Can you work these out from the drawing? Everything is in mm from the part's minimum corner. Coordinates: 2 decimals unless noted, no trailing zeros. Loops run counter-clockwise (first coordinate to the right, second up) from the corner with the lowest first, then second, coordinate; pieces in that order, holes last.
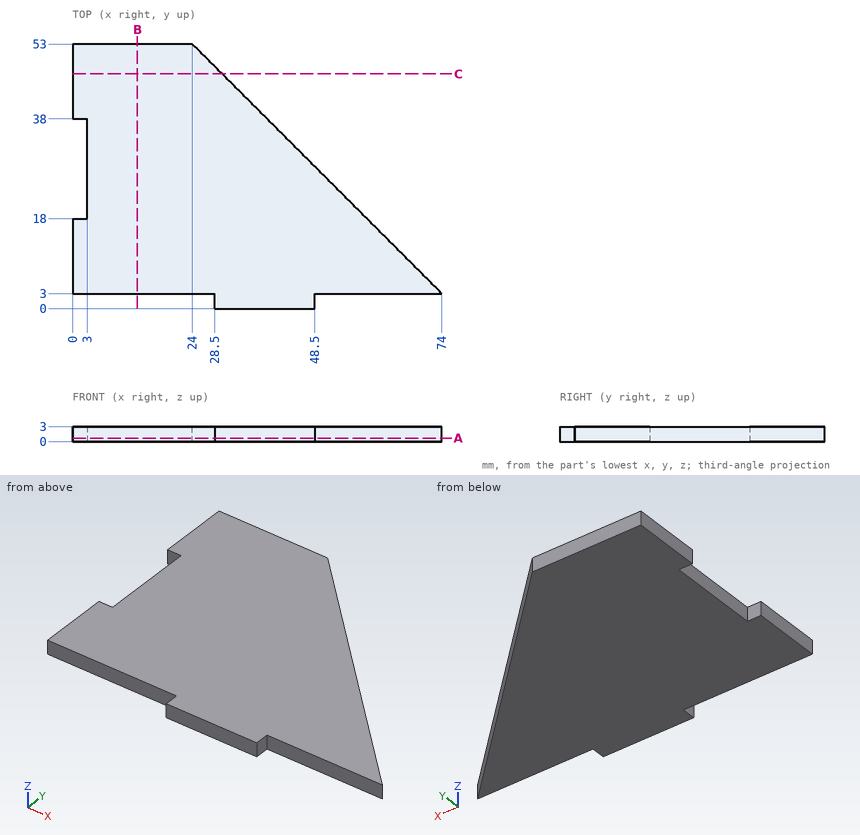
Item 1: Suppose I cut it at B-B, the plane x = 13. Please give me the cut outline in (y, z).
Results are:
outline: (3, 0) - (53, 0) - (53, 3) - (3, 3) - close
Item 2: Suppose I cut it at C-C, the plane y = 47. Please give me the cut outline in (x, z).
Results are:
outline: (0, 0) - (30, 0) - (30, 3) - (0, 3) - close
Item 3: Suppose I cut it at A-A, the plane z = 0.7. Please give me the cut outline in (x, y).
Results are:
outline: (0, 3) - (28.5, 3) - (28.5, 0) - (48.5, 0) - (48.5, 3) - (74, 3) - (24, 53) - (0, 53) - (0, 38) - (3, 38) - (3, 18) - (0, 18) - close
Item 4: I need wall thicknesses on line 1 along Y through (x, z) = (22, 0.8); line 2 along X through (y, z) = (2, 1.5); line 3 along X through (y, z) = (42, 2.4). Which ranges of each line are inside material? Lowest first, please.
Results are:
line 1: y = 3 to 53
line 2: x = 28.5 to 48.5
line 3: x = 0 to 35
Item 5: I'm going to push flat-ended pins straight in: P1, Ø1.5, axis at x = 1.5, z = 1, coming from the -Y side; P2, Ø1, axis at x = 46, z = 2, coming from the +Y side. Where does each tip first touch, or does it pass through?
Results are:
P1: stops at y = 3
P2: stops at y = 31.5
